```python
from build123d import *

# Parameters (mm, degrees)
F0_R     = 11.125
F1_DEPTH = 7
F2_R     = 2
F3_R     = 2


with BuildPart() as f1:
    # F0 (on Top) → F1 (new body)
    with BuildSketch(Plane.XY):
        with BuildLine():
            ThreePointArc((18.74733, 10.826125), (13.90015, 10.191447), (9.27886, 11.785701))
            ThreePointArc((9.27886, 11.785701), (0, 15), (-9.27886, 11.785701))
            ThreePointArc((-9.27886, 11.785701), (-13.90015, 10.191447), (-18.74733, 10.826125))
            ThreePointArc((-18.74733, 10.826125), (-36.951446, 0), (-18.74733, -10.826125))
            ThreePointArc((-18.74733, -10.826125), (-13.90015, -10.191447), (-9.27886, -11.785701))
            ThreePointArc((-9.27886, -11.785701), (0, -15), (9.27886, -11.785701))
            ThreePointArc((9.27886, -11.785701), (13.90015, -10.191447), (18.74733, -10.826125))
            ThreePointArc((18.74733, -10.826125), (36.951446, 0), (18.74733, 10.826125))
        make_face()
        Polygon((-29.725315, 8.825), (-19.535083, 8.825), (-14.439967, 0), (-19.535083, -8.825), (-29.725315, -8.825), (-34.820431, 0), align=None, mode=Mode.SUBTRACT)
        Circle(F0_R, mode=Mode.SUBTRACT)
        Polygon((14.439967, 0), (19.535083, 8.825), (29.725315, 8.825), (34.820431, 0), (29.725315, -8.825), (19.535083, -8.825), align=None, mode=Mode.SUBTRACT)
    extrude(amount=F1_DEPTH)

    # F2
    f2_edges = [f1.edges().sort_by_distance(p)[0] for p in [
        (-36.951446, 0, 7),
        (-13.90015, -10.191447, 7),
        (0, -15, 7),
        (13.90015, -10.191447, 7),
        (36.951446, 0, 7),
        (13.90015, 10.191447, 7),
        (0, 15, 7),
        (-13.90015, 10.191447, 7),
    ]]
    fillet(f2_edges, radius=F2_R)

    # F3
    f3_edges = [f1.edges().sort_by_distance(p)[0] for p in [
        (-13.90015, -10.191447, 0),
        (-36.951446, 0, 0),
        (-13.90015, 10.191447, 0),
        (0, 15, 0),
        (13.90015, 10.191447, 0),
        (36.951446, 0, 0),
        (13.90015, -10.191447, 0),
        (0, -15, 0),
    ]]
    fillet(f3_edges, radius=F3_R)


solid = f1.part
```
Source: CAD feature listing. Evaluate the final solid. Frame: model axes, mm. A direction names the side the tool comes from. Coordinates: 2 decimals unless noted, no trailing zeros. Loops run counter-clockwise (first coordinate to the right, second up) from the corner with the lowest first, then second, coordinate; pieces in that order, holes last. Notation, with made-up numbers: (76, 78.5) -> (108, 78.5) arc R18 cw to (108, 90.5) -> close; hole circle Ø11 at (83.5, 30). An arc over 180 degrees is marked (long way). One line per item, written item: value. Start each with the question number.
Q1. Section query A-A, the plane x = 0. Return the cut outline in (y, z) (3 decimals), and give its area (3 significant figures).
Q2. Set-up query: faces 1 (the face through (32.24, 4.47, 3.45)), 2 (the face through (-11, 4, 7)). Return all of +Z, -Z, +X, -X, +Y, -Y with unobstructed straight access to the full face (end or side cutting, diameter ignored); none if empty.
Q3. Section query B-B, the plane z = 1.25. Give the number of separate pieces and of enclosed holes in the cut face, and give its area (3 significant figures).
Q4. Line query: line 1 along X through (y, z) = (-1, 2.25); line 2 along Y through (x, z) = (0, 3.25) (3 decimals); line 3 along X through (y, z) = (-7, 2). Output: solid intervals per line, ascending.
Q5. Mould query, pull axis X, two halves, no side actions, for faces 3 (the face through (-11, 4, 0)), 4 (the face through (17.02, -4.47, 3.45)). Classes: pulls with the +X half, pulls with the -X half, needs draft (parallel to the pull), parting line crosses it, or undercut.
Q6. Contact query for flat-ended pins moving along their axis: P1, Ø2, axis at x = -25.5, z = 2.5, coming from the +Y side; P2, Ø4, axis at x = -4.5, z = 5.5, coming from the -Y side; P3, Ø1.5, axis at y = 10, z = 3, coming from the +X side. Output: stop coordinate, or through.
Results:
1. outline: (-15, 2) arc R2 ccw to (-13, 0) -> (-11.125, 0) -> (-11.125, 7) -> (-13, 7) arc R2 ccw to (-15, 5) -> close; (11.125, 0) -> (13, 0) arc R2 ccw to (15, 2) -> (15, 5) arc R2 ccw to (13, 7) -> (11.125, 7) -> close
1. area: 50.8 mm^2
2. face 1: +Z, -Z
2. face 2: +Z, +X, -X, +Y, -Y
3. separate pieces: 1
3. enclosed holes: 3
3. area: 719 mm^2
4. line 1: -36.91 to -34.24, -15.02 to -11.08, 11.08 to 15.02, 34.24 to 36.91
4. line 2: -15 to -11.125, 11.125 to 15
4. line 3: -34.77 to -30.78, -18.48 to -8.65, 8.65 to 18.48, 30.78 to 34.77
5. face 3: needs draft
5. face 4: undercut
6. P1: y = 12.32
6. P2: y = -14.78
6. P3: x = 32.77
